Read the model definition and answer for the solid it produces. Units are mm, in the model's axes. Face numbers are marked on the shaded views. A direction names the side the tool comes from. Round coordinates to 2 decimals unless told otherwise and drop trailing zeros. Order: outer loops, then holes, each group sorted by start corner. A loop starts at its lowest first (then second) coordinate and runs counter-clockwise, first axis right, second up. Notation, with made-up numbers: (69, -37.75) -> (81, -37.75) arc R12 ccw to (81, -21.75) -> close; hole circle Ø7 at (-32, -20). An arc over 180 degrees is marked (long way). Use a Markdown table: item, result. Add a question column.
1. Section A-A, the plane z = 5.5 is taken. Give the vertices of the cut face in (x, y).
2. For the marked faces 4, 5, 6, 7 and 8, determine the directions among +Z, -Z, +X, -X, +Y, -Y from which every point of the face is accessible in a straight line to the end or side of a thin tool.
3. Consider L1, parallel to Y at x = -8.8, z = 6; L2, parallel to Y at x = -9.4, z = 8.75; L3, parallel to X at y = -4.5, z = 5.25. Determine where each line is inside the solid, lowest interval first. Write a range as [from, to].
4. Section C-C, the plane y = -2 is taken. Give the vertices of the cut face in (x, z), then the cut area to 4 significant figures.
5. Section D-D, the plane z = 4.25 is taken. Give the vertices of the cut face in (x, y).
6. Given pin 1 (0.5 mm diameter, centred on x = -5, y = -3, fed in from +Z); pin 2 (1 mm diameter, centred on x = -7, y = -4.5, fed in from +Z); pin 3 (3 mm diameter, centred on x = -7, z = 7, fed in from -Y), each flat-ended and moving along its own axis, determine where each tip first touches the part or whether it passes through.
7. The mould has two halves that part along X. Classify the marked faces 1, 2 and 3: +X half, -X half, draft (parallel to the pull), parting line (faces both ways), or undercut.
8. Section B-B, the plane x = -6.2 is taken. Give the vertices of the cut face in (y, z), then the cut area to 3 significant figures.
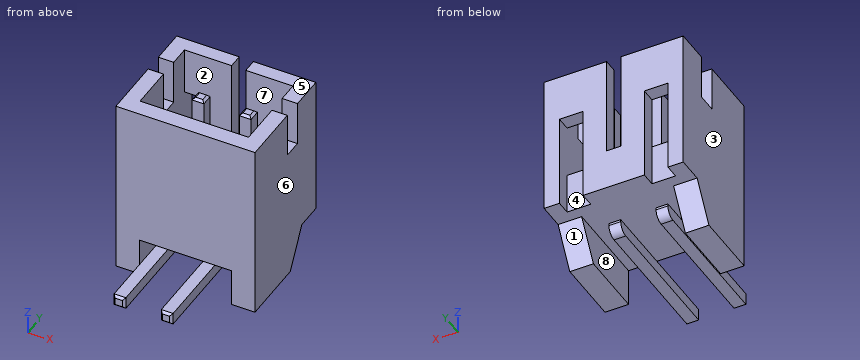
```python
from build123d import *

# Parameters (mm, degrees)
EXTRUDE_1_DEPTH     = 0.6
EXTRUDE_2_DEPTH     = 3.5
SKETCH_3_W          = 5.9
SKETCH_3_H          = 6
EXTRUDE_3_DEPTH     = 0.7
EXTRUDE_4_REACH     = 15.883
SKETCH_4_W          = 0.5
SKETCH_4_H          = 2.85
SKETCH_5_W          = 0.5
SKETCH_5_H          = 0.5
EXTRUDE_5_DEPTH     = 3.4
EXTRUDE_6_REACH     = 17.656
SKETCH_7_W          = 0.5
SKETCH_7_H          = 2.85
SKETCH_8_W          = 0.5
SKETCH_8_H          = 0.5
EXTRUDE_7_DEPTH     = 3.4
SKETCH_9_W          = 4.6
SKETCH_9_H          = 1.85
CUT_EXTRUDE_1_DEPTH = 0.6
CUT_EXTRUDE_2_REACH = 16.257
SKETCH_10_W         = 1.9
SKETCH_10_H         = 0.8
SKETCH_11_W         = 1.9
SKETCH_11_H         = 0.8
CUT_EXTRUDE_3_DEPTH = 15.257366517
SKETCH_12_W         = 1
SKETCH_12_H         = 3.7
EXTRUDE_8_DEPTH     = 1.6
SKETCH_13_W         = 1
SKETCH_13_H         = 3.7
EXTRUDE_9_DEPTH     = 1.6
SKETCH_14_W         = 0.5
SKETCH_14_H         = 0.5
EXTRUDE_10_DEPTH    = 3.3
SKETCH_15_W         = 0.5
SKETCH_15_H         = 0.5
EXTRUDE_11_DEPTH    = 3.3
DRAFT_1_ANGLE       = 45
DRAFT_2_ANGLE       = 30
FILLET_1_R          = 0.4
CHAMFER_1_SIZE      = 0.1


with BuildPart() as part:
    # 草图1 → 凸台-拉伸1 (new body)
    with BuildSketch(Plane.XZ.offset(1.8)):
        Polygon((-7.45, 8.95), (-7.45, 4.7), (-8.05, 4.7), (-8.05, 8.95), (-10.7, 8.95), (-10.7, 2.95), (-10.05, 2.95), (-10.05, 6.95), (-9.05, 6.95), (-9.05, 2.95), (-6.45, 2.95), (-6.45, 6.95), (-5.45, 6.95), (-5.45, 2.95), (-4.8, 2.95), (-4.8, 8.95), align=None)
    extrude(amount=-EXTRUDE_1_DEPTH)

    # 草图2 → 凸台-拉伸2 (add)
    with BuildSketch(Plane.XZ.offset(1.8)):
        Polygon((-10.7, 8.95), (-10.05, 8.95), (-10.05, 4.7), (-5.45, 4.7), (-5.45, 8.95), (-4.8, 8.95), (-4.8, 2.95), (-10.7, 2.95), align=None)
    extrude(amount=EXTRUDE_2_DEPTH)

    # 草图3 → 凸台-拉伸3 (add)
    with BuildSketch(Plane.XZ.offset(5.3)):
        with Locations((-7.75, 5.95)):
            Rectangle(SKETCH_3_W, SKETCH_3_H)
    extrude(amount=EXTRUDE_3_DEPTH)

    # 草图4 → 凸台-拉伸4 (add, up to next)
    with BuildSketch(Plane(origin=(0, 0, 2.45), x_dir=(-1, 0, 0), z_dir=(0, 0, -1)), mode=Mode.PRIVATE) as extrude_4_sk1:
        with Locations((8.75, -4.575)):
            Rectangle(SKETCH_4_W, SKETCH_4_H)
    extrude_4_tool1 = extrude(extrude_4_sk1.sketch, amount=-EXTRUDE_4_REACH, mode=Mode.PRIVATE) - part.part
    add(extrude_4_tool1.solids().sort_by_distance((-8.75, -4.575, 2.45))[0])

    # 草图5 → 凸台-拉伸5 (add)
    with BuildSketch(Plane.XZ.offset(6)):
        with Locations((-8.75, 2.7)):
            Rectangle(SKETCH_5_W, SKETCH_5_H)
    extrude(amount=EXTRUDE_5_DEPTH)

    # 草图7 → 凸台-拉伸6 (add, up to next)
    with BuildSketch(Plane(origin=(0, 0, 2.45), x_dir=(-1, 0, 0), z_dir=(0, 0, -1)), mode=Mode.PRIVATE) as extrude_6_sk1:
        with Locations((6.75, -4.575)):
            Rectangle(SKETCH_7_W, SKETCH_7_H)
    extrude_6_tool1 = extrude(extrude_6_sk1.sketch, amount=-EXTRUDE_6_REACH, mode=Mode.PRIVATE) - part.part
    add(extrude_6_tool1.solids().sort_by_distance((-6.75, -4.575, 2.45))[0])

    # 草图8 → 凸台-拉伸7 (add)
    with BuildSketch(Plane.XZ.offset(6)):
        with Locations((-6.75, 2.7)):
            Rectangle(SKETCH_8_W, SKETCH_8_H)
    extrude(amount=EXTRUDE_7_DEPTH)

    # 草图9 → 切除-拉伸1 (cut)
    with BuildSketch(Plane.XY.offset(4.7)):
        with Locations((-7.75, -4.375)):
            Rectangle(SKETCH_9_W, SKETCH_9_H)
    extrude(amount=-CUT_EXTRUDE_1_DEPTH, mode=Mode.SUBTRACT)

    # 草图10 → 切除-拉伸2 (cut, up to next)
    with BuildSketch(Plane.ZY.offset(10.7), mode=Mode.PRIVATE) as cut_extrude_2_sk1:
        with Locations((8, -3.05)):
            Rectangle(SKETCH_10_W, SKETCH_10_H)
    cut_extrude_2_tool1 = extrude(cut_extrude_2_sk1.sketch, amount=-CUT_EXTRUDE_2_REACH, mode=Mode.PRIVATE) & part.part
    add(cut_extrude_2_tool1.solids().sort_by_distance((-10.7, -3.05, 8))[0], mode=Mode.SUBTRACT)

    # 草图11 → 切除-拉伸3 (cut, through all)
    with BuildSketch(Plane(origin=(-4.8, 0, 0), x_dir=(0, 0, -1), z_dir=(1, 0, 0))):
        with Locations((-8, -3.05)):
            Rectangle(SKETCH_11_W, SKETCH_11_H)
    extrude(amount=-CUT_EXTRUDE_3_DEPTH, mode=Mode.SUBTRACT)

    # 草图12 → 凸台-拉伸8 (add)
    with BuildSketch(Plane(origin=(0, 0, 2.95), x_dir=(-1, 0, 0), z_dir=(0, 0, -1))):
        with Locations((10.2, -4.15)):
            Rectangle(SKETCH_12_W, SKETCH_12_H)
    extrude(amount=EXTRUDE_8_DEPTH)

    # 草图13 → 凸台-拉伸9 (add)
    with BuildSketch(Plane(origin=(0, 0, 2.95), x_dir=(-1, 0, 0), z_dir=(0, 0, -1))):
        with Locations((5.3, -4.15)):
            Rectangle(SKETCH_13_W, SKETCH_13_H)
    extrude(amount=EXTRUDE_9_DEPTH)

    # 草图14 → 凸台-拉伸10 (add)
    with BuildSketch(Plane.XY.offset(4.7)):
        with Locations((-6.75, -2.9)):
            Rectangle(SKETCH_14_W, SKETCH_14_H)
    extrude(amount=EXTRUDE_10_DEPTH)

    # 草图15 → 凸台-拉伸11 (add)
    with BuildSketch(Plane.XY.offset(4.7)):
        with Locations((-8.75, -2.9)):
            Rectangle(SKETCH_15_W, SKETCH_15_H)
    extrude(amount=EXTRUDE_11_DEPTH)

    # 拔模1
    draft_1_faces = [part.faces().sort_by_distance(p)[0] for p in [
        (-7.75, -3.45, 4.4),
    ]]
    draft(draft_1_faces, Plane(origin=(-7.45, -1.2, 4.7), x_dir=(0, 1, 0), z_dir=(0, 0, 1)), DRAFT_1_ANGLE)

    # 拔模2
    draft_2_faces = [part.faces().sort_by_distance(p)[0] for p in [
        (-5.3, -2.3, 2.15),
        (-10.2, -2.3, 2.15),
    ]]
    draft(draft_2_faces, Plane(origin=(-5.45, -1.2, 2.95), x_dir=(-1, 0, 0), z_dir=(0, 0, -1)), DRAFT_2_ANGLE)

    # 圆角1
    fillet_1_edges = [part.edges().sort_by_distance(p)[0] for p in [
        (-8.75, -3.15, 2.45),
        (-6.75, -3.15, 2.45),
    ]]
    fillet(fillet_1_edges, radius=FILLET_1_R)

    # 倒角1
    chamfer_1_edges = [part.edges().sort_by_distance(p)[0] for p in [
        (-6.75, -9.4, 2.95),
        (-6.5, -9.4, 2.7),
        (-6.75, -9.4, 2.45),
        (-7, -9.4, 2.7),
        (-8.75, -9.4, 2.95),
        (-8.5, -9.4, 2.7),
        (-8.75, -9.4, 2.45),
        (-9, -9.4, 2.7),
        (-6.75, -2.65, 8),
        (-6.5, -2.9, 8),
        (-6.75, -3.15, 8),
        (-7, -2.9, 8),
        (-8.75, -2.65, 8),
        (-8.5, -2.9, 8),
        (-8.75, -3.15, 8),
        (-9, -2.9, 8),
    ]]
    chamfer(chamfer_1_edges, length=CHAMFER_1_SIZE)


solid = part.part
```
Verdict:
| question | item | result |
|---|---|---|
| 1 | outline | (-10.7, -6) -> (-4.8, -6) -> (-4.8, -1.2) -> (-5.45, -1.2) -> (-5.45, -5.3) -> (-10.05, -5.3) -> (-10.05, -1.2) -> (-10.7, -1.2) -> close; (-9.05, -1.8) -> (-8.05, -1.8) -> (-8.05, -1.2) -> (-9.05, -1.2) -> close; (-9, -3.15) -> (-8.5, -3.15) -> (-8.5, -2.65) -> (-9, -2.65) -> close; (-7.45, -1.8) -> (-6.45, -1.8) -> (-6.45, -1.2) -> (-7.45, -1.2) -> close; (-7, -3.15) -> (-6.5, -3.15) -> (-6.5, -2.65) -> (-7, -2.65) -> close |
| 2 | face 4 | -Z, +Y |
| 2 | face 5 | +Z, +X, -X, +Y, -Y |
| 2 | face 6 | +Z, -Z, +X, +Y, -Y |
| 2 | face 7 | +Z |
| 2 | face 8 | -Z, +Y, -Y |
| 3 | L1 | y = [-6, -5.3], [-3.15, -2.65], [-1.8, -1.2] |
| 3 | L2 | y = [-6, -5.3], [-1.8, -1.2] |
| 3 | L3 | x = [-10.7, -10.05], [-5.45, -4.8] |
| 4 | outline | (-10.7, 2.95) -> (-4.8, 2.95) -> (-4.8, 8.95) -> (-5.45, 8.95) -> (-5.45, 4.7) -> (-10.05, 4.7) -> (-10.05, 8.95) -> (-10.7, 8.95) -> close |
| 4 | area | 15.85 mm2 |
| 5 | outline | (-10.7, -6) -> (-4.8, -6) -> (-4.8, -1.2) -> (-5.45, -1.2) -> (-5.45, -1.8) -> (-6.45, -1.8) -> (-6.45, -1.2) -> (-9.05, -1.2) -> (-9.05, -1.8) -> (-10.05, -1.8) -> (-10.05, -1.2) -> (-10.7, -1.2) -> close; hole (-10.05, -5.3) -> (-5.45, -5.3) -> (-5.45, -3.9) -> (-10.05, -3.9) -> close |
| 6 | pin 1 | stops at z = 7.05 |
| 6 | pin 2 | stops at z = 4.15 |
| 6 | pin 3 | stops at y = -6 |
| 7 | face 1 | draft |
| 7 | face 2 | undercut |
| 7 | face 3 | -X half |
| 8 | outline | (-6, 2.95) -> (-1.8, 2.95) -> (-1.8, 4.7) -> (-3.45, 4.7) -> (-4.05, 4.1) -> (-5.3, 4.1) -> (-5.3, 8.95) -> (-6, 8.95) -> close; (-1.8, 6.95) -> (-1.2, 6.95) -> (-1.2, 8.95) -> (-1.8, 8.95) -> close |
| 8 | area | 10.6 mm2 |
